from build123d import *

# Parameters (mm, degrees)
SKETCH1_W           = 52
SKETCH1_H           = 25
BOSS_EXTRUDE1_DEPTH = 2
SKETCH2_W           = 4
SKETCH2_H           = 25
BOSS_EXTRUDE2_DEPTH = 20
FILLET1_R           = 3
SKETCH4_R           = 1.725
CUT_EXTRUDE2_DEPTH  = 2
SKETCH5_W           = 48
SKETCH5_H           = 2.5
BOSS_EXTRUDE3_DEPTH = 2.5
SKETCH6_W           = 20
SKETCH6_H           = 14
CUT_EXTRUDE3_DEPTH  = 2


with BuildPart() as part:
    # Sketch1 → Boss-Extrude1 (new body)
    with BuildSketch(Plane.XY):
        with Locations((26, -12.5)):
            Rectangle(SKETCH1_W, SKETCH1_H)
    extrude(amount=BOSS_EXTRUDE1_DEPTH)

    # Sketch2 → Boss-Extrude2 (add)
    with BuildSketch(Plane(origin=(0, 0, 2), x_dir=(-1, 0, 0), z_dir=(0, 0, -1))):
        with Locations((-50, -12.5)):
            Rectangle(SKETCH2_W, SKETCH2_H)
    extrude(amount=-BOSS_EXTRUDE2_DEPTH)

    # Fillet1
    fillet1_edges = [part.edges().sort_by_distance(p)[0] for p in [
        (50, -25, 22),
        (50, 0, 22),
    ]]
    fillet(fillet1_edges, radius=FILLET1_R)

    # Sketch4 → Cut-Extrude2 (cut)
    with BuildSketch(Plane.XY.offset(2)):
        with Locations((41.277695867, -12.5)):
            Circle(SKETCH4_R)
        with Locations((6.277695867, -12.5)):
            Circle(SKETCH4_R)
    extrude(amount=-CUT_EXTRUDE2_DEPTH, mode=Mode.SUBTRACT)

    # Sketch5 → Boss-Extrude3 (add)
    with BuildSketch(Plane(origin=(0, 0, 2), x_dir=(-1, 0, 0), z_dir=(0, 0, -1))):
        with Locations((-24, -23.75)):
            Rectangle(SKETCH5_W, SKETCH5_H)
        with Locations((-24, -1.25)):
            Rectangle(SKETCH5_W, SKETCH5_H)
    extrude(amount=-BOSS_EXTRUDE3_DEPTH)

    # Sketch6 → Cut-Extrude3 (cut)
    with BuildSketch(Plane.XY.offset(2)):
        with Locations((23.277695867, -12.531043961)):
            Rectangle(SKETCH6_W, SKETCH6_H)
    extrude(amount=-CUT_EXTRUDE3_DEPTH, mode=Mode.SUBTRACT)


solid = part.part
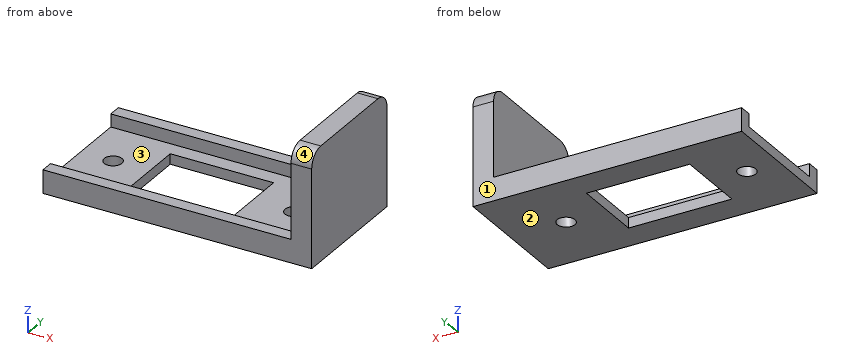
Can you work these out from the model? Positions are in its coordinate system, mm. Face numbers are marked on the shaded views. Coordinates: 2 decimals unless noted, no trailing zeros. Write each loop counter-clockwise with the first axis right and the second up, starting at its lowest first coordinate (ties: lowest second). Pieces come first, ordered by that corner, then holes.
Q1. Imagine slicing it at A-A, the plane y = -16.75. List the corners of the cut face in (x, z) for me, plus the area to 3 significant figures.
Results found:
outline: (0, 0) - (13.28, 0) - (13.28, 2) - (0, 2) - close; (33.28, 0) - (52, 0) - (52, 22) - (48, 22) - (48, 2) - (33.28, 2) - close
area: 144 mm2
Q2. Imagine slicing it at D-D, the plane z = 2.5. List the corners of the cut face in (x, y) for me.
Results found:
outline: (0, -25) - (52, -25) - (52, 0) - (0, 0) - (0, -2.5) - (48, -2.5) - (48, -22.5) - (0, -22.5) - close
Q3. Imagine slicing it at B-B, the plane y = -12.5. List the corners of the cut face in (x, z) for me, plus the area to 3 significant figures.
Results found:
outline: (0, 0) - (4.55, 0) - (4.55, 2) - (0, 2) - close; (8, 0) - (13.28, 0) - (13.28, 2) - (8, 2) - close; (33.28, 0) - (39.55, 0) - (39.55, 2) - (33.28, 2) - close; (43, 0) - (52, 0) - (52, 22) - (48, 22) - (48, 2) - (43, 2) - close
area: 130 mm2
Q4. For P1, Ø1.5, axis at y = -9.5, z = 15, coming from the -X side; P2, Ø2, axis at x = 34.5, y = -1, coming from the +Z side; P3, Ø10, axis at x = 29.5, y = -14.5, coming from the +Z side; P4, Ø8, axis at x = 19.5, z = 6.5, coming from the -Y side, each with a flat end and sliding along its axis, tell me the tip position at first contact or that it passes through.
Results found:
P1: stops at x = 48
P2: stops at z = 4.5
P3: stops at z = 2
P4: stops at y = -25
Q5. If we mould it in two halves opening along Y, with no side actions, what happens to the marked faces 1, 2, 3 and 4? For each: +Y half, -Y half, draft (parallel to the pull), parting line (faces both ways), or undercut.
Results found:
face 1: +Y half
face 2: draft
face 3: undercut
face 4: -Y half
Q6. Please list where these lines run through material, in increasing order: L1, parallel to Z at x = 35, y = -18.5; L2, parallel to X at y = -13, z = 10.5; L3, parallel to Z at x = 49, y = -23.
Results found:
L1: z = 0 to 2
L2: x = 48 to 52
L3: z = 0 to 21.83
Q7. Imagine slicing it at C-C, the plane x = 14.5. List the corners of the cut face in (y, z) for me, plus the area to 3 significant figures.
Results found:
outline: (-25, 0) - (-19.53, 0) - (-19.53, 2) - (-22.5, 2) - (-22.5, 4.5) - (-25, 4.5) - close; (-5.53, 0) - (0, 0) - (0, 4.5) - (-2.5, 4.5) - (-2.5, 2) - (-5.53, 2) - close
area: 34.5 mm2
